```python
from build123d import *

# Parameters (mm, degrees)
SKETCH_1_W                   = 42
SKETCH_1_H                   = 16
EXTRUDE_1_DEPTH              = 10
CUT_EXTRUDE_1_DEPTH          = 47.043457733
SKETCH_4_W                   = 15.7
SKETCH_4_H                   = 16
CUT_EXTRUDE_2_DEPTH          = 5
HOLE_WIZARD_M3_1_D           = 3.6
HOLE_WIZARD_M3_1_CBORE_D     = 6.5
HOLE_WIZARD_M3_1_CBORE_DEPTH = 3


with BuildPart() as part:
    # 草图1 → 凸台-拉伸1 (new body)
    with BuildSketch(Plane.XY):
        with Locations((21, 8)):
            Rectangle(SKETCH_1_W, SKETCH_1_H)
    extrude(amount=EXTRUDE_1_DEPTH)

    # 草图2 → 切除-拉伸1 (cut, through all)
    with BuildSketch(Plane.XY.offset(10)):
        Polygon((28.75, 12), (13.25, 12), (13.25, 4), (14.65, 4), (14.65, 6), (27.35, 6), (27.35, 4), (28.75, 4), align=None)
    extrude(amount=-CUT_EXTRUDE_1_DEPTH, mode=Mode.SUBTRACT)

    # 草图4 → 切除-拉伸2 (cut)
    with BuildSketch(Plane.XY.offset(10)):
        with Locations((21, 8)):
            Rectangle(SKETCH_4_W, SKETCH_4_H)
    extrude(amount=-CUT_EXTRUDE_2_DEPTH, mode=Mode.SUBTRACT)

    # M3 六角凹头螺钉的柱形沉头孔1 (through all)
    with Locations(Plane(origin=(0, 0, 0), x_dir=(-1, 0, 0), z_dir=(0, 0, -1))):
        with Locations((-38, 8), (-4, 8)):
            CounterBoreHole(HOLE_WIZARD_M3_1_D / 2, HOLE_WIZARD_M3_1_CBORE_D / 2, HOLE_WIZARD_M3_1_CBORE_DEPTH)


solid = part.part
```
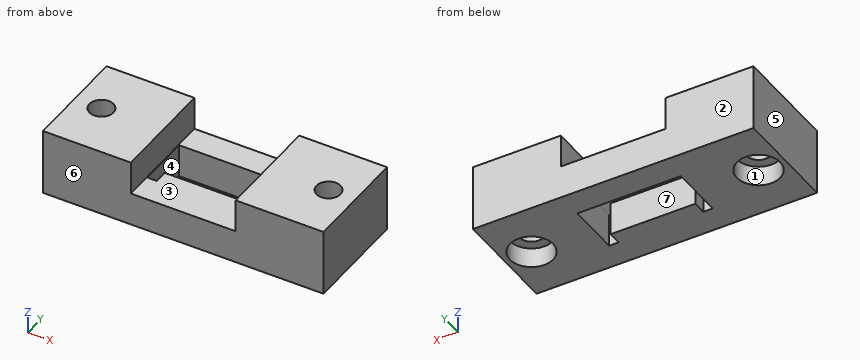
Work out the finished part from the listing and answer in its coordinate system (mm). Face numbers are marked on the shaded views. A direction names the side the tool comes from. Give positions to 0.01 mm unless a question says otherwise; leave off trailing zeros. Write each loop counter-clockwise with the first axis right and the second up, starting at its lowest first coordinate (ties: lowest second). Pieces come first, ordered by that corner, then holes.
(1) Flat-ended cylindrical pins translate along their axes: pin 1 Ø4 at (x, y) = (4, 8) entering from -Z; pin 2 Ø4.5 at (x, y) = (18.5, 10.5) entering from +Z. Find the tip coordinate at first contact, or state that the pin passes through.
Final values:
pin 1: stops at z = 3
pin 2: stops at z = 5
(2) The part is cut by section C-C on y = 8. Write down the section's boundary in (x, z), plus the area to 3 significant figures.
Final values:
outline: (0, 0) - (0.75, 0) - (0.75, 3) - (2.2, 3) - (2.2, 10) - (0, 10) - close; (5.8, 3) - (7.25, 3) - (7.25, 0) - (13.25, 0) - (13.25, 5) - (13.15, 5) - (13.15, 10) - (5.8, 10) - close; (28.75, 0) - (34.75, 0) - (34.75, 3) - (36.2, 3) - (36.2, 10) - (28.85, 10) - (28.85, 5) - (28.75, 5) - close; (39.8, 3) - (41.25, 3) - (41.25, 0) - (42, 0) - (42, 10) - (39.8, 10) - close
area: 175 mm2
(3) The part is cut by section A-A on z = 7.25. Write down the section's boundary in (x, y).
Final values:
outline: (0, 0) - (13.15, 0) - (13.15, 16) - (0, 16) - close; (28.85, 0) - (42, 0) - (42, 16) - (28.85, 16) - close; hole circle Ø3.6 at (4, 8); hole circle Ø3.6 at (38, 8)
(4) The part is cut by section D-D on z = 4. Write down the section's boundary in (x, y).
Final values:
outline: (0, 0) - (42, 0) - (42, 16) - (0, 16) - close; hole circle Ø3.6 at (4, 8); hole (13.25, 4) - (14.65, 4) - (14.65, 6) - (27.35, 6) - (27.35, 4) - (28.75, 4) - (28.75, 12) - (13.25, 12) - close; hole circle Ø3.6 at (38, 8)
(5) The part is cut by section B-B on x = 26. Write down the section's boundary in (y, z).
Final values:
outline: (0, 0) - (6, 0) - (6, 5) - (0, 5) - close; (12, 0) - (16, 0) - (16, 5) - (12, 5) - close
(6) Straight lines are drawn through the part: line 1 (X direction, y = 7.75, z = 1); line 2 (Y direction, x = 38, z = 1.2); line 3 (Y direction, x = 25, z = 1.5). For each, find the intervals that lie inside material, in ascending order.
Final values:
line 1: x = 0 to 0.76, 7.24 to 13.25, 28.75 to 34.76, 41.24 to 42
line 2: y = 0 to 4.75, 11.25 to 16
line 3: y = 0 to 6, 12 to 16
(7) Which of the six approach directions +Z, -Z, +X, -X, +Y, -Y give full straight-line access (tool end or side, diameter ignored) to the marked faces 1, 2, 3 and 4?
Final values:
face 1: -Z
face 2: +Z, -Z, +X, -X, +Y
face 3: +Z, +Y, -Y
face 4: +Z, -Z
(8) The mould has two halves that part along Y. Classify the marked faces 5, 6 and 7: pulls with the +Y half, pulls with the -Y half, needs draft (parallel to the pull), parting line crosses it, or undercut.
Final values:
face 5: needs draft
face 6: pulls with the -Y half
face 7: undercut
